```python
from build123d import *

# Parameters (mm, degrees)
F1_DEPTH    = 7
F2_R        = 2
F3_DEPTH    = 4.2
F4_DEPTH    = 25
F5_R        = 2.5
F6_DEPTH    = 25
F7_R        = 8
F8_R        = 5
F9_T1_DEPTH = 52
F11_DEPTH   = 25
F13_DEPTH   = 25
F14_R       = 3
F15_DEPTH   = 25
F16_R       = 7


# Not quite as in the source:
# - a fillet or chamfer that OpenCascade refuses, or shapes differently, is made with other operations: its cross-section is extruded or revolved along the edge and cut away or added
# - ends of sketch curves that miss each other by under 0.0002 mm in the source are joined
# - a feature names something its author has since deleted; it is built from what else it names


with BuildPart() as f1:
    # F0 (on Top) → F1 (new body)
    with BuildSketch(Plane.XY):
        Polygon((-2, 17), (-17.0000004771, 17), (-16.9999997194, -10.0000004771), (17.0000002806, -9.9999995229), (17, 4.771e-07), (16.9999997755, 8), (-2, 8), align=None)
        with BuildLine():
            Line((17, 4.771e-07), (17.0000002806, -9.9999995229))
            Line((17.0000002806, -9.9999995229), (65.7550022822, -9.9999995229))
            ThreePointArc((65.7550022822, -9.9999995229), (64.0000002806, -4.9999995229), (65.7550022822, 4.771e-07))
            Line((65.7550022822, 4.771e-07), (17, 4.771e-07))
        make_face()
        with BuildLine():
            ThreePointArc((65.7550022822, 4.771e-07), (64.0000002806, -4.9999995229), (65.7550022822, -9.9999995229))
            Line((65.7550022822, -9.9999995229), (72.0000002806, -9.9999995229))
            Line((72.0000002806, -9.9999995229), (72.0000002806, 4.771e-07))
            Line((72.0000002806, 4.771e-07), (65.7550022822, 4.771e-07))
        make_face()
        with BuildLine():
            Line((72.0000002806, -9.9999995229), (65.7550022822, -9.9999995229))
            ThreePointArc((65.7550022822, -9.9999995229), (74.6495300514, -12.5485087793), (80.0000002806, -4.9999995229))
            ThreePointArc((80.0000002806, -4.9999995229), (74.6495300514, 2.5485097334), (65.7550022822, 4.771e-07))
            Line((65.7550022822, 4.771e-07), (72.0000002806, 4.771e-07))
            Line((72.0000002806, 4.771e-07), (72.0000002806, -9.9999995229))
        make_face()
    extrude(amount=F1_DEPTH)

    # F2 (on face) → F3 (cut)
    with BuildSketch(Plane.XY.offset(7)):
        Polygon((11.5, 8), (-2, 8), (-3.4079101854, -0.8891950654), (10.0920898146, -0.8891950654), align=None)
        with Locations((4.0460449073, 3.5554024673)):
            Circle(F2_R, mode=Mode.SUBTRACT)
    extrude(amount=-F3_DEPTH, mode=Mode.SUBTRACT)

    # F4 (cut): a face of the model
    f4_faces = [f1.faces().sort_by_distance(p)[0] for p in [
        (4.0460449073, 3.5554024673, 7),
    ]]
    extrude(f4_faces, amount=-F4_DEPTH, mode=Mode.SUBTRACT)

    # F5 (on face) → F6 (cut)
    with BuildSketch(Plane.XY.offset(7)):
        with Locations((-9, 5)):
            Circle(F5_R)
    extrude(amount=-F6_DEPTH, mode=Mode.SUBTRACT)

    # F7
    f7_edges = [f1.edges().sort_by_distance(p)[0] for p in [
        (-17, 17, 3.5),
    ]]
    fillet(f7_edges, radius=F7_R)

    # F8
    f8_edges = [f1.edges().sort_by_distance(p)[0] for p in [
        (-17, -10, 3.5),
    ]]
    fillet(f8_edges, radius=F8_R)

    # F9: fillet of radius 9 on 1 edges, made by hand

    # F9_s2 → F9_t1 (cut)
    with BuildSketch(Plane.XY.offset(-22.5)):
        with BuildLine():
            ThreePointArc((-11, 17), (-4.6360389693, 14.3639610307), (-2, 8))
            Line((-2, 8), (-2, 17))
            Line((-2, 17), (-11, 17))
        make_face()
    extrude(amount=F9_T1_DEPTH, mode=Mode.SUBTRACT)

    # F10 (on face) → F11 (cut)
    with BuildSketch(Plane.XY.offset(7)):
        with BuildLine():
            ThreePointArc((-3.2, 12.4899888642), (-2.3051739523, 10.3237900078), (-2, 8))
            Line((-2, 8), (-2, 18))
            Line((-2, 18), (-3.2, 18))
            Line((-3.2, 18), (-3.2, 12.4899888642))
        make_face()
        with BuildLine():
            Line((-3.2, 8), (-2, 8))
            ThreePointArc((-2, 8), (-2.3051739523, 10.3237900078), (-3.2, 12.4899888642))
            Line((-3.2, 12.4899888642), (-3.2, 8))
        make_face()
    extrude(amount=-F11_DEPTH, mode=Mode.SUBTRACT)

    # F12 (on face) → F13 (cut)
    with BuildSketch(Plane.XY.offset(7)):
        with BuildLine():
            ThreePointArc((-17, 4.9999997208), (-11.9664795245, 12.4296701966), (-3.2, 10.5099909256))
            Line((-3.2, 10.5099909256), (-3.2, 12.4899888642))
            ThreePointArc((-3.2, 12.4899888642), (-6.0560248177, 15.5204460903), (-9.9704600393, 16.9409198335))
            ThreePointArc((-9.9704600393, 16.9409198335), (-14.9901454961, 14.3026559347), (-17.0000002526, 8.9999997755))
            Line((-17.0000002526, 8.9999997755), (-17, 4.9999997208))
        make_face()
    extrude(amount=-F13_DEPTH, mode=Mode.SUBTRACT)

    # F14 (on face) → F15 (cut)
    with BuildSketch(Plane.XY.offset(7)):
        with Locations((72.0000002806, -4.9999995229)):
            Circle(F14_R)
    extrude(amount=-F15_DEPTH, mode=Mode.SUBTRACT)

    # F16
    f16_edges = [f1.edges().sort_by_distance(p)[0] for p in [
        (17, 0, 3.5),
        (65.755002, -10, 3.5),
        (65.755002, 0, 3.5),
    ]]
    fillet(f16_edges, radius=F16_R)


solid = f1.part
```
Source: CAD feature listing. Evaluate the final solid. Frame: model axes, mm. A direction names the side the tool comes from. Round coordinates to 2 decimals unless told otherwise and drop trailing zeros. Loops run counter-clockwise (first coordinate to the right, second up) from the corner with the lowest first, then second, coordinate; pieces in that order, holes last.
(1) Access query for faces 4 (the flat face through (10.786, 3.493, 4.929)), 5 (the flat face through (7, 8, 2)), 6 (the cylindrical face through (65.18, 0.35, 3.55)). Directions: +Z, -Z, +X, -X, +Y, -Y. A direction counts if a zero-diameter tool reaches every point of the face in a straight line with its end or side. Return the directions, or none.
From the geometry:
face 4: +Z, +Y
face 5: +Z, -Z, +X, +Y
face 6: +Z, -Z, +Y
(2) Section query D-D (z = 1.5). Output: boundary loops of the cut face in (x, y).
From the geometry:
outline: (-17, -5) arc R5 ccw to (-12, -10) - (63, -10) arc R7 cw to (67.2, -11.4) arc R8 ccw (long way) to (67.2, 1.4) arc R7 cw to (63, 0) - (24, 0) arc R7 cw to (17, 7) - (17, 8) - (-3.2, 8) - (-3.2, 10.51) arc R8 ccw to (-17, 5) - close; hole circle Ø5 at (-9, 5); hole circle Ø4 at (4.05, 3.56); hole circle Ø6 at (72, -5)
(3) Pull-direction query (Y, two-part tool) for faces 1 (the cylindrical face through (69.6, -6.8, 3.5)), 2 (the cylindrical face through (-16, -8, 4)), 3 (the cylindrical face through (19, 2.1, 3.5)); classes: +Y half, -Y half, draft (parallel to the pull), parting line (faces both ways), or undercut.
From the geometry:
face 1: undercut
face 2: -Y half
face 3: +Y half
(4) Contact query for flat-ended pins moving along their axis: pin 1 Ø1.3 at (x, z) = (1.5, 4.5) entering from +Y; pin 2 Ø5 at (x, y) = (4.05, 3.56) entering from +Z; pin 3 Ø1.5 at (y, z) = (-2.5, 6) entering from +X. Output: stop coordinate, or through.
From the geometry:
pin 1: stops at y = -0.89
pin 2: stops at z = 2.8
pin 3: stops at x = 79.81
(5) Material intervals for probe 1 along X at (y, z) = (-4.75, 2.25); probe 2 along X at (y, z) = (0.75, 4.5); probe 3 along Y at (x, z) = (29, 4.25), sorted ascending.
From the geometry:
probe 1: x = -17 to 69.01, 74.99 to 80
probe 2: x = -17 to -3.15, 10.35 to 20.85, 66.15 to 77.56
probe 3: y = -10 to 0
(6) Section query B-B (z = 5.25). Output: boundary loops of the cut face in (x, y), and give its area (3 significant figures).
From the geometry:
outline: (-17, -5) arc R5 ccw to (-12, -10) - (63, -10) arc R7 cw to (67.2, -11.4) arc R8 ccw (long way) to (67.2, 1.4) arc R7 cw to (63, 0) - (24, 0) arc R7 cw to (17, 7) - (17, 8) - (11.5, 8) - (10.09, -0.89) - (-3.41, -0.89) - (-2, 8) - (-3.2, 8) - (-3.2, 10.51) arc R8 ccw to (-17, 5) - close; hole circle Ø5 at (-9, 5); hole circle Ø6 at (72, -5)
area: 1,180 mm2
(7) Section query A-A (x = 72). Output: boundary loops of the cut face in (y, z).
From the geometry:
outline: (-13, 0) - (-8, 0) - (-8, 7) - (-13, 7) - close; (-2, 0) - (3, 0) - (3, 7) - (-2, 7) - close
(8) Section query C-C (y = -6.5). Output: boundary loops of the cut face in (x, z), and give its area (3 significant figures).
From the geometry:
outline: (-16.77, 0) - (69.4, 0) - (69.4, 7) - (-16.77, 7) - close; (74.6, 0) - (79.86, 0) - (79.86, 7) - (74.6, 7) - close
area: 640 mm2
